Can you work these out from the model? Positions are in its coordinate system, mm. Face numbers are marked on the shaded views. A direction names the side the tool comes from. Give positions to 0.01 mm unless a question says otherwise; leave off trailing zeros. Loops run counter-clockwise (first coordinate to the right, second up) from the corner with the lowest first, then second, coordinate; pieces in that order, holes last. Notation, with made-up numbers: (-21, 37) -> (-13, 37) arc R9 cw to (-13, 49) -> close; hole circle Ø10 at (-15, -37). An arc over 180 degrees is marked (long way). Use CSV: the item, a comma, the result in double quotes.
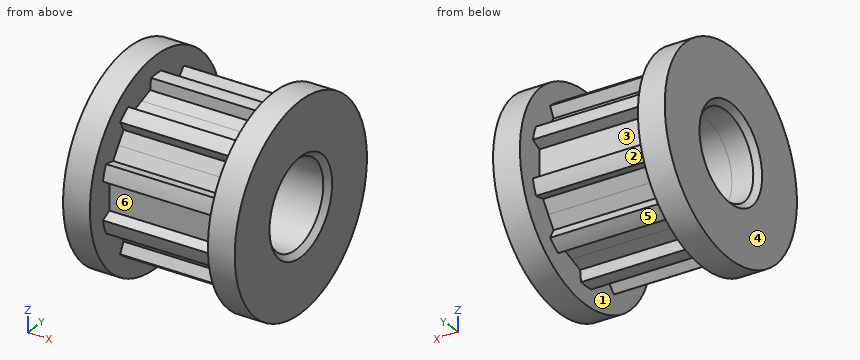
from build123d import *

# Parameters (mm, degrees)
SKETCH_1_R      = 4
EXTRUDE_1_DEPTH = 11
SKETCH_2_R      = 9.5
SKETCH_2_R_2    = 4
EXTRUDE_2_DEPTH = 2.5
SKETCH_3_R      = 9.5
SKETCH_3_R_2    = 4
EXTRUDE_3_DEPTH = 2.5
CHAMFER_1_SIZE  = 0.5


with BuildPart() as part:
    # 草图1 → 凸台-拉伸1 (new body)
    with BuildSketch(Plane(origin=(0, 0, 0), x_dir=(0, 0, -1), z_dir=(1, 0, 0))):
        with BuildLine():
            Line((1.728321742, 7.636871346), (1.29, 6.696887337))
            Line((1.29, 6.696887337), (0, 6.696887337))
            Line((0, 6.696887337), (-1.29, 6.696887337))
            Line((-1.29, 6.696887337), (-1.728321742, 7.636871346))
            ThreePointArc((-1.728321742, 7.636871346), (-2.419603066, 7.446772523), (-3.09059869, 7.194240734))
            Line((-3.09059869, 7.194240734), (-2.89269969, 6.17613864))
            Line((-2.89269969, 6.17613864), (-3.936331613, 5.417895665))
            Line((-3.936331613, 5.417895665), (-4.979963536, 4.659652689))
            Line((-4.979963536, 4.659652689), (-5.887082012, 5.162476672))
            ThreePointArc((-5.887082012, 5.162476672), (-6.334603066, 4.602358525), (-6.729015468, 4.003654685))
            Line((-6.729015468, 4.003654685), (-5.970486418, 3.296314902))
            Line((-5.970486418, 3.296314902), (-6.36911834, 2.069451996))
            Line((-6.36911834, 2.069451996), (-6.767750263, 0.84258909))
            Line((-6.767750263, 0.84258909), (-7.797177048, 0.716191375))
            ThreePointArc((-7.797177048, 0.716191375), (-7.83, 0), (-7.797177048, -0.716191375))
            Line((-7.797177048, -0.716191375), (-6.767750263, -0.84258909))
            Line((-6.767750263, -0.84258909), (-6.36911834, -2.069451996))
            Line((-6.36911834, -2.069451996), (-5.970486418, -3.296314902))
            Line((-5.970486418, -3.296314902), (-6.729015468, -4.003654685))
            ThreePointArc((-6.729015468, -4.003654685), (-6.334603066, -4.602358525), (-5.887082012, -5.162476672))
            Line((-5.887082012, -5.162476672), (-4.979963536, -4.659652689))
            Line((-4.979963536, -4.659652689), (-3.936331613, -5.417895665))
            Line((-3.936331613, -5.417895665), (-2.89269969, -6.17613864))
            Line((-2.89269969, -6.17613864), (-3.09059869, -7.194240734))
            ThreePointArc((-3.09059869, -7.194240734), (-2.419603066, -7.446772523), (-1.728321742, -7.636871346))
            Line((-1.728321742, -7.636871346), (-1.29, -6.696887337))
            Line((-1.29, -6.696887337), (0, -6.696887337))
            Line((0, -6.696887337), (1.29, -6.696887337))
            Line((1.29, -6.696887337), (1.728321742, -7.636871346))
            ThreePointArc((1.728321742, -7.636871346), (2.419603066, -7.446772523), (3.09059869, -7.194240734))
            Line((3.09059869, -7.194240734), (2.89269969, -6.17613864))
            Line((2.89269969, -6.17613864), (3.936331613, -5.417895665))
            Line((3.936331613, -5.417895665), (4.979963536, -4.659652689))
            Line((4.979963536, -4.659652689), (5.887082012, -5.162476672))
            ThreePointArc((5.887082012, -5.162476672), (6.334603066, -4.602358525), (6.729015468, -4.003654685))
            Line((6.729015468, -4.003654685), (5.970486418, -3.296314902))
            Line((5.970486418, -3.296314902), (6.36911834, -2.069451996))
            Line((6.36911834, -2.069451996), (6.767750263, -0.84258909))
            Line((6.767750263, -0.84258909), (7.797177048, -0.716191375))
            ThreePointArc((7.797177048, -0.716191375), (7.83, 0), (7.797177048, 0.716191375))
            Line((7.797177048, 0.716191375), (6.767750263, 0.84258909))
            Line((6.767750263, 0.84258909), (6.36911834, 2.069451996))
            Line((6.36911834, 2.069451996), (5.970486418, 3.296314902))
            Line((5.970486418, 3.296314902), (6.729015468, 4.003654685))
            ThreePointArc((6.729015468, 4.003654685), (6.334603066, 4.602358525), (5.887082012, 5.162476672))
            Line((5.887082012, 5.162476672), (4.979963536, 4.659652689))
            Line((4.979963536, 4.659652689), (3.936331613, 5.417895665))
            Line((3.936331613, 5.417895665), (2.89269969, 6.17613864))
            Line((2.89269969, 6.17613864), (3.09059869, 7.194240734))
            ThreePointArc((3.09059869, 7.194240734), (2.419603066, 7.446772523), (1.728321742, 7.636871346))
        make_face()
        Circle(SKETCH_1_R, mode=Mode.SUBTRACT)
    extrude(amount=EXTRUDE_1_DEPTH)

    # 草图2 → 凸台-拉伸2 (add)
    with BuildSketch(Plane(origin=(11, 0, 0), x_dir=(0, 0, -1), z_dir=(1, 0, 0))):
        Circle(SKETCH_2_R)
        Circle(SKETCH_2_R_2, mode=Mode.SUBTRACT)
    extrude(amount=EXTRUDE_2_DEPTH)

    # 草图3 → 凸台-拉伸3 (add)
    with BuildSketch(Plane.ZY):
        Circle(SKETCH_3_R)
        Circle(SKETCH_3_R_2, mode=Mode.SUBTRACT)
    extrude(amount=EXTRUDE_3_DEPTH)

    # 倒角1
    chamfer_1_edges = [part.edges().sort_by_distance(p)[0] for p in [
        (13.5, 0, 4),
        (-2.5, 0, -4),
    ]]
    chamfer(chamfer_1_edges, length=CHAMFER_1_SIZE)


solid = part.part
(1) If I drill on L1, parallel to Y at x = -0.9, z = 0; L2, parallel to X at y = 8.25, z = -4; L3, parallel to Y at x = 10.5, z = 0, over which ranges is the centre line in solid material (lowest first)? Write a range as from..to.
Answer sheet:
L1,"y = -9.5..-4, 4..9.5"
L2,"x = -2.5..0, 11..13.5"
L3,"y = -6.7..-4, 4..6.7"
(2) Will these pins go through, and if not, where does the flat tip stop? pin 1 Ø3 at (x, z) = (8.5, -6) entering from -Y; pin 2 Ø5 at (x, y) = (6, 1) entering from -Z; pin 3 Ø1 at (x, z) = (3, -0.5) entering from +Y; pin 4 Ø5 at (y, z) = (0, 0) entering from -X.
Answer sheet:
pin 1,"stops at y = -5.16"
pin 2,"stops at z = -7.83"
pin 3,"stops at y = 6.7"
pin 4,"passes through"
(3) Which directions (+Z, -Z, +X, -X, +Y, -Y) give clear straight access to the entire face, cutting with the end or side of a thin tool? Please do the marked faces 1, 2 and 3.
Answer sheet:
face 1,"none"
face 2,"-Z, +Y"
face 3,"+Y"
(4) We'd pull the mould along Z, two halves only. Please class the marked faces 4, 5 and 6: released by +Z, released by -Z, zero draft, split by the parting line, or undercut.
Answer sheet:
face 4,"zero draft"
face 5,"released by -Z"
face 6,"undercut"
(5) If we section it at B-B, the plane y = 0: Write out the boundary of the cut face in (x, z), then the cut area to 3 significant figures.
Answer sheet:
outline,"(-2.5, -9.5) -> (0, -9.5) -> (0, -7.83) -> (11, -7.83) -> (11, -9.5) -> (13.5, -9.5) -> (13.5, -4.5) -> (13, -4) -> (-2, -4) -> (-2.5, -4.5) -> close; (-2.5, 4.5) -> (-2, 4) -> (13, 4) -> (13.5, 4.5) -> (13.5, 9.5) -> (11, 9.5) -> (11, 7.83) -> (0, 7.83) -> (0, 9.5) -> (-2.5, 9.5) -> close"
area,"139 mm2"
(6) If we section it at A-A, the plane z = 0: Write out the boundary of the cut face in (x, y), then the cut area to 3 significant figures.
Answer sheet:
outline,"(-2.5, -9.5) -> (0, -9.5) -> (0, -6.7) -> (11, -6.7) -> (11, -9.5) -> (13.5, -9.5) -> (13.5, -4.5) -> (13, -4) -> (-2, -4) -> (-2.5, -4.5) -> close; (-2.5, 4.5) -> (-2, 4) -> (13, 4) -> (13.5, 4.5) -> (13.5, 9.5) -> (11, 9.5) -> (11, 6.7) -> (0, 6.7) -> (0, 9.5) -> (-2.5, 9.5) -> close"
area,"114 mm2"
(7) If we section it at D-D, the plane x = 11.5: Write out the boundary of the cut face in (y, z), then the cut area to 3 significant figures.
Answer sheet:
outline,"circle Ø19 at (0, 0); hole circle Ø8 at (0, 0)"
area,"233 mm2"
(8) If we section it at C-C, the plane z = -5.5: Write out the boundary of the cut face in (x, y).
Answer sheet:
outline,"(-2.5, -7.75) -> (0, -7.75) -> (0, -4.95) -> (11, -4.95) -> (11, -7.75) -> (13.5, -7.75) -> (13.5, 7.75) -> (11, 7.75) -> (11, 4.95) -> (0, 4.95) -> (0, 7.75) -> (-2.5, 7.75) -> close"
